For this review, take the finished solid that the model builds, in its own axes (mm). A direction names the side the tool comes from. Give positions to 0.01 mm unless a question says otherwise; leave off trailing zeros. Loops run counter-clockwise (first coordinate to the right, second up) from the corner with the lowest first, then second, coordinate; pieces in that order, holes last.
```python
from build123d import *

# Parameters (mm, degrees)
CHAMFER1_SIZE  = 0.4
EXTRUDE1_START = -3.25
SKETCH2_R      = 11.925743973
EXTRUDE1_DEPTH = 3.25
EXTRUDE2_START = -8.8
SKETCH3_R      = 13.491172398
EXTRUDE2_DEPTH = 8.8


with BuildPart() as part:
    # Sketch1 → Revolve1 (revolve)
    with BuildSketch(Plane.XY, mode=Mode.PRIVATE) as revolve1_sk:
        Polygon((0, 0), (0, 5), (1.5, 5), (1.5, 6.275), (11, 6.275), (11, 8), (10.5, 8), (10.5, 11), (19.3, 11), (19.3, 6.5), (20.3, 6.5), (20.3, 8.4), (24.65, 8.4), (24.65, 10.75), (27.9, 10.75), (27.9, 3.82), (40, 3.82), (40, 2.3), (38, 2.3), (38, 1.6), (12, 1.6), (12, 0), align=None)
    revolve(revolve1_sk.sketch.rotate(Axis((0, 0, 0), (1, 0, 0)), 90), axis=Axis((0, 0, 0), (1, 0, 0)))

    # Chamfer1
    chamfer1_edges = [part.edges().sort_by_distance(p)[0] for p in [
        (40, 0, -3.82),
    ]]
    chamfer(chamfer1_edges, length=CHAMFER1_SIZE)

    # Sketch2 → Extrude1 (cut)
    with BuildSketch(Plane(origin=(27.9, 0, 0), x_dir=(0, 0, -1), z_dir=(1, 0, 0)).offset(EXTRUDE1_START)):
        Circle(SKETCH2_R)
        Polygon((0, 10.75), (-9.309773091, 5.375), (-9.309773091, -5.375), (0, -10.75), (9.309773091, -5.375), (9.309773091, 5.375), align=None, mode=Mode.SUBTRACT)
    extrude(amount=EXTRUDE1_DEPTH, mode=Mode.SUBTRACT)

    # Sketch3 → Extrude2 (cut)
    with BuildSketch(Plane(origin=(19.3, 0, 0), x_dir=(0, 0, -1), z_dir=(1, 0, 0)).offset(EXTRUDE2_START)):
        Circle(SKETCH3_R)
        Polygon((-5.5, 9.526279442), (-11, 0), (-5.5, -9.526279442), (5.5, -9.526279442), (11, 0), (5.5, 9.526279442), align=None, mode=Mode.SUBTRACT)
    extrude(amount=EXTRUDE2_DEPTH, mode=Mode.SUBTRACT)


solid = part.part
```
Item 1: Tool access review of faces 4 (the flat face through (10.5, -6, -6)), 5 (the cylindrical face through (24.818, -0.481, 1.526)), 6 (the flat face through (26, 0, -9.31)), 7 (the flat face through (14.838, 4.696, -8.288)): name each direction out of +Z, -Z, +X, -X, +Y, -Y from which nothing blocks a thin tool from reaching the whole face with its end or side.
Answer:
face 4: -X
face 5: +X
face 6: -Z, +X, +Y, -Y
face 7: -Z, -X, +Y
Item 2: Clearance check with flat-ended pins moving along their axes: pin 1 Ø4 at (y, z) = (-3.5, 6.5) entering from -X; pin 2 Ø1.5 at (x, z) = (29.5, 8) entering from +Y; pin 3 Ø3.5 at (y, z) = (0, 0.5) entering from +X; pin 4 Ø3.5 at (x, y) = (26.5, 0.5) entering from +Z. State where each tip first meets the part, or that it passes through.
Answer:
pin 1: stops at x = 1.5
pin 2: passes through
pin 3: stops at x = 38
pin 4: stops at z = 9.31
Item 3: Take a section at C-C on z = 4.5. Give the boundary of the cut face in (x, y), and give its area (3 significant figures).
Answer:
outline: (0, -2.18) - (1.5, -2.18) - (1.5, -4.37) - (11, -4.37) - (11, -6.61) - (10.5, -6.61) - (10.5, -9.53) - (19.3, -9.53) - (19.3, -4.69) - (20.3, -4.69) - (20.3, -7.09) - (24.65, -7.09) - (24.65, -8.15) - (27.9, -8.15) - (27.9, 8.15) - (24.65, 8.15) - (24.65, 7.09) - (20.3, 7.09) - (20.3, 4.69) - (19.3, 4.69) - (19.3, 9.53) - (10.5, 9.53) - (10.5, 6.61) - (11, 6.61) - (11, 4.37) - (1.5, 4.37) - (1.5, 2.18) - (0, 2.18) - close
area: 375 mm2
Item 4: For L1, parallel to Y at x = 10.85, z = 0 (3 decimals); L2, parallel to X at y = -2.25, z = -9; L3, parallel to Y at x = 39.05, z = 0, list the stretches that pass through material, from the lowest coordinate up.
Answer:
L1: y = -9.526 to -8, -6.275 to 6.275, 8 to 9.526
L2: x = 10.5 to 19.3, 24.65 to 27.9
L3: y = -3.82 to -2.3, 2.3 to 3.82
Item 5: Take a section at D-D on x = 3. Give the boundary of the cut face in (y, z) (3 decimals).
Answer:
outline: circle Ø12.55 at (0, 0)
Item 6: The part is to be moulded in two halves that separate along Y. For faces 1 (the flat face through (11, 3.5, 5.4)), 2 (the flat face through (26.25, -8.1, -4.59)), 3 (the flat face through (19.3, -6.5, 2.3)), say which applies: released by +Y, released by -Y, zero draft, split by the parting line, or undercut.
Answer:
face 1: undercut
face 2: released by -Y
face 3: zero draft
Item 7: Take a section at B-B on x = 36. Give the boundary of the cut face in (y, z), and give its area (3 significant figures).
Answer:
outline: circle Ø7.64 at (0, 0); hole circle Ø3.2 at (0, 0)
area: 37.8 mm2
Item 8: Take a section at A-A on y = 7. Give the boundary of the cut face in (x, z).
Answer:
outline: (10.5, -6.96) - (19.3, -6.96) - (19.3, 6.96) - (10.5, 6.96) - (10.5, 3.87) - (11, 3.87) - (11, -3.87) - (10.5, -3.87) - close; (20.3, -4.64) - (24.65, -4.64) - (24.65, -6.5) - (27.9, -6.5) - (27.9, 6.5) - (24.65, 6.5) - (24.65, 4.64) - (20.3, 4.64) - close
